Design review of the part shown in the three views and the two pictorial views. Dimensions are in mm from the part's minimum x, y and z. A direction names the side the tool comes from. Round coordinates to 2 decimals unless told otherwise and drop trailing zeros. Loops run counter-clockwise (first coordinate to the right, second up) from the corner with the lowest first, then second, coordinate; pieces in that order, holes last. Notation, with made-up numbers: (30.5, 82.25) - (42.5, 82.25) arc R26 cw to (42.5, 100.25) - close; hole circle Ø7 at (-13.75, -3.5). An arc over 180 degrees is marked (long way). Return JSON: item names as keys, results as strings. Group by question number.
(1) We need section B-B, the plane y = 13.25. Write out the cut boundary in (x, z).
(2) Wall thickness on L1, parallel to Z at x = 47, y = 7.5 (1 decimal); L2, parallel to X at y = 9, z = 13; L3, parallel to X at y = 12, z = 4.25 (1 decimal): over which ranges is each line inside the solid? List them lowest first. Write a range as [from, to].
(3) We need section D-D, the plane x = 40. Write out the cut boundary in (y, z), and give its area (3 significant figures).
(4) We need section C-C, the plane z = 7. Write out the cut boundary in (x, y), and give its area (3 significant figures).
(5) For the marked faces 4, 5 and 6, list the 3-axis set-ups (+Z, -Z, +X, -X, +Y, -Y) from which the entire face can be reached by the end or side of a thin tool; tool diameter is ignored.
(6) The part is to be moulded in two halves that separate along X. For the marked faces 1, 2 and 3, say which applies: pulls with the +X half, pulls with the -X half, needs draft (parallel to the pull), parting line crosses it, or undercut.
(7) Clearance check with flat-ended pins moving along their axes: pin 1 (6 mm diameter, centred on x = 47, z = 11, fed in from -Y) (1 decimal); pin 2 (5 mm diameter, centred on x = 47.5, z = 3, fed in from -Y); pin 3 (6 mm diameter, centred on x = 4, z = 10.5, fed in from -Y). State where each tip first meets the part, or that it passes through.
(8) We need section A-A, the plane z = 3. Write out the cut boundary in (x, y), and give its area (3 significant figures).
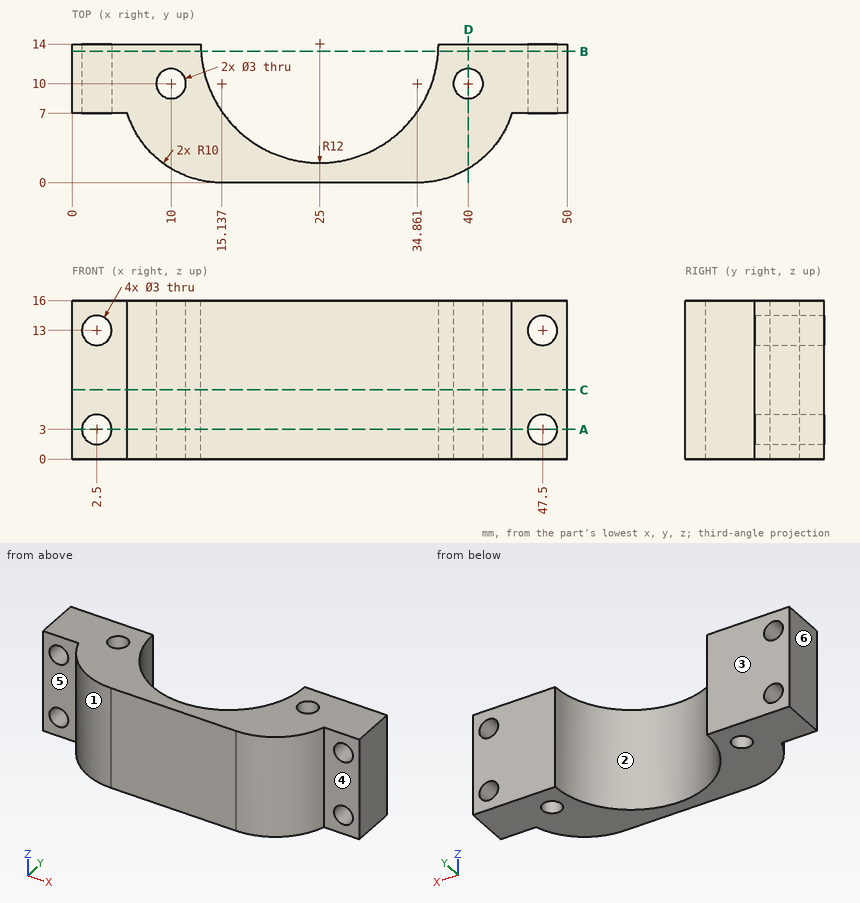
Solutions:
{
 "1": {"outline": "(0, 0) - (13.02, 0) - (13.02, 16) - (0, 16) - close; (36.98, 0) - (50, 0) - (50, 16) - (36.98, 16) - close; hole circle Ø3 at (2.5, 3); hole circle Ø3 at (2.5, 13); hole circle Ø3 at (47.5, 3); hole circle Ø3 at (47.5, 13)"},
 "2": {"L1": "[0, 1.6], [4.4, 11.6], [14.4, 16]", "L2": "[0, 1], [4, 8.88], [11.12, 14.09], [35.91, 38.88], [41.12, 46], [49, 50]", "L3": "[0, 1.7], [3.3, 13.2], [36.8, 46.7], [48.3, 50]"},
 "3": {"outline": "(1.42, 0) - (8.5, 0) - (8.5, 16) - (1.42, 16) - close; (11.5, 0) - (14, 0) - (14, 16) - (11.5, 16) - close", "area": "153 mm^2"},
 "4": {"outline": "(0, 7) - (5.6, 7) arc R10 ccw to (15.14, 0) - (34.86, 0) arc R10 ccw to (44.4, 7) - (50, 7) - (50, 14) - (37, 14) arc R12 cw to (13, 14) - (0, 14) - close; hole circle Ø3 at (10, 10); hole circle Ø3 at (40, 10)", "area": "346 mm^2"},
 "5": {"face 4": "+Z, -Z, +X, -Y", "face 5": "+Z, -Z, -X, -Y", "face 6": "+Z, -Z, -X, +Y, -Y"},
 "6": {"face 1": "pulls with the -X half", "face 2": "undercut", "face 3": "needs draft"},
 "7": {"pin 1": "y = 5.9", "pin 2": "y = 7", "pin 3": "y = 4.19"},
 "8": {"outline": "(0, 7) - (1, 7) - (1, 14) - (0, 14) - close; (4, 7) - (5.6, 7) arc R10 ccw to (15.14, 0) - (34.86, 0) arc R10 ccw to (44.4, 7) - (46, 7) - (46, 14) - (37, 14) arc R12 cw to (13, 14) - (4, 14) - close; (49, 7) - (50, 7) - (50, 14) - (49, 14) - close; hole circle Ø3 at (10, 10); hole circle Ø3 at (40, 10)", "area": "304 mm^2"}
}
